Input: part model. Units: mm. Frame: model coordinates. Face numbers are marked on the shaded views. A direction names the side the tool comes from. Coordinates: 2 decimals unless noted, no trailing zeros. Loops run counter-clockwise (first coordinate to the right, second up) from the corner with the lowest first, then second, coordinate; pieces in that order, holes last. Notation, with made-up numbers: (9, -24.75) - (26, -24.75) arc R19 ccw to (26, 11.25) - close; hole circle Ø8 at (71, -20.5). An arc over 180 degrees is marked (long way). Use one line per item in the form item = value.
from build123d import *

# Parameters (mm, degrees)
CHAMFER1_SIZE      = 2
CHAMFER2_SIZE      = 1
CUT_EXTRUDE1_DEPTH = 8
CHAMFER3_SIZE      = 1
SKETCH4_R          = 4
CUT_EXTRUDE2_DEPTH = 39


with BuildPart() as part:
    # Sketch1 → Revolve1 (revolve)
    with BuildSketch(Plane.XY):
        Polygon((0, 0), (0, 12), (16, 12), (16, 7.981), (46, 7.981), (46, 0), align=None)
    revolve(axis=Axis((-88.705490849, 0, 0), (1, 0, 0)))

    # Chamfer1
    chamfer1_edges = [part.edges().sort_by_distance(p)[0] for p in [
        (46, -7.981, 0),
    ]]
    chamfer(chamfer1_edges, length=CHAMFER1_SIZE)

    # Chamfer2
    chamfer2_edges = [part.edges().sort_by_distance(p)[0] for p in [
        (0, -12, 0),
    ]]
    chamfer(chamfer2_edges, length=CHAMFER2_SIZE)

    # Sketch3 → Cut-Extrude1 (cut)
    with BuildSketch(Plane(origin=(0, 0, 0), x_dir=(0, 0, -1), z_dir=(1, 0, 0))):
        Polygon((-8.082903769, 0), (-4.041451884, -7), (4.041451884, -7), (8.082903769, 0), (4.041451884, 7), (-4.041451884, 7), align=None)
    extrude(amount=CUT_EXTRUDE1_DEPTH, mode=Mode.SUBTRACT)

    # Chamfer3
    chamfer3_edges = [part.edges().sort_by_distance(p)[0] for p in [
        (0, 3.5, 6.062177826),
        (0, -3.5, 6.062177826),
        (0, -7, 0),
        (0, -3.5, -6.062177826),
        (0, 3.5, -6.062177826),
        (0, 7, 0),
    ]]
    chamfer(chamfer3_edges, length=CHAMFER3_SIZE)

    # Sketch4 → Cut-Extrude2 (cut, through all)
    with BuildSketch(Plane.ZY.offset(-8)):
        Circle(SKETCH4_R)
    extrude(amount=-CUT_EXTRUDE2_DEPTH, mode=Mode.SUBTRACT)


solid = part.part
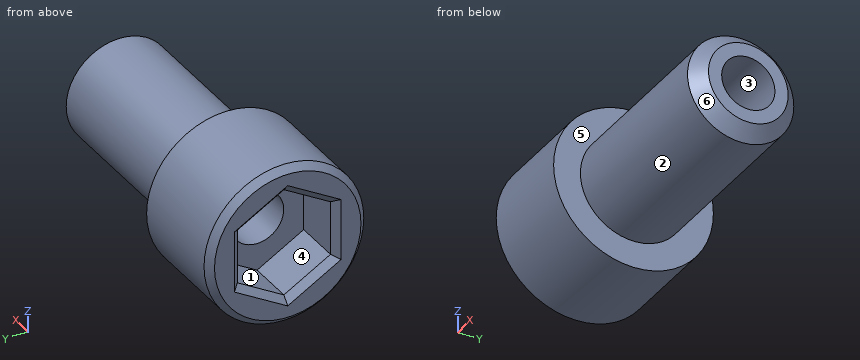
Q1. Pull-direction query (Y, two-part tool) for the marked faces 4, 5 and 6; classes: pulls with the +Y half, pulls with the -Y half, needs draft (parallel to the pull), parting line crosses it, or undercut.
Check values:
face_4 = undercut
face_5 = needs draft
face_6 = parting line crosses it
Q2. First-contact query: P1, Ø3.5, axis at x = 5, z = 1.5, coming from the -Y side; P2, Ø7, axis at y = 1.5, z = -2, coming from the -X side; P3, Ø4, axis at x = 36, z = 3, coming from the +Y side; P4, Ø1.5, axis at x = 35.5, y = -6, coming from the -Z side. Flat tips, straight axial feed; report the tip coordinate or a pass-through.
Check values:
P1 = -12
P2 = 8
P3 = 7.92
P4 = -6.01
Q3. Cut plane A-A, the plane z = 0. Return loops of the section in (x, y), then the cut area to 3 significant figures.
Check values:
outline = (0, -11) - (1, -12) - (16, -12) - (16, -7.98) - (44, -7.98) - (46, -5.98) - (46, -4) - (8, -4) - (8, -7) - (1, -7) - (0, -8) - close; (0, 8) - (1, 7) - (8, 7) - (8, 4) - (46, 4) - (46, 5.98) - (44, 7.98) - (16, 7.98) - (16, 12) - (1, 12) - (0, 11) - close
area = 441 mm²
Q4. Cut plane B-B, the plane x = 19.5. Return loops of the section in (y, z), then the cut area to 3 significant figures.
Check values:
outline = circle Ø15.96 at (0, 0); hole circle Ø8 at (0, 0)
area = 150 mm²
Q5. Ray query, line 1 along X through (y, z) = (-3.25, -8); line 2 along Y through (x, z) = (14.5, 2.5); line 3 along Z through (x, y) = (36.5, -3). Return the intervals inside material, ascending. Write a range as [from, to].
Check values:
line_1 = [0, 16]
line_2 = [-11.74, -3.12], [3.12, 11.74]
line_3 = [-7.4, -2.65], [2.65, 7.4]
Q6. Set-up query: the marked faces 1, 2 and 3. Return all of +Z, -Z, +X, -X, +Y, -Y with unobstructed straight access to the full face (end or side cutting, diameter ignored); none if empty.
Check values:
face_1 = -X
face_2 = +X
face_3 = +X, -X
